Job drawing, mm, ordinate dimensions from the low corner. One solid piece. Give positions to 0.01 mm unless a question says otherwise; leave off trailing zeros. Write each loop counter-clockwise with the first axis right and the second up, starting at its lowest first coordinate (ties: lowest second). Pieces come first, ordered by that corner, then holes. Notation, with made-up numbers: M 49.5,-39 L 92.5,-39 A20 cw 92.5,-21 Z; hole C 58.5,86.25 d3. An arc over 180 degrees is marked long. Answer as CSV lines item,"result". Start each with the question number.
Item 1: Band-saw the part on B-B, the plane x = 21.5. List the corners of the cut face in (y, z).
Item 2: Band-saw the part on A-A, the plane z = 10.5. List the corners of the cut face in (x, y), then the cut area to 3 significant figures.
Item 3: Wall check: L1, parallel to Y at x = 44.5, z = 16.5; L2, parallel to Y at x = 37.5, z = 32; L3, parallel to Z at x = 46, y = 27. Give the ranges that are in metal, low to high. Write a range as from..to.
Item 4: Band-saw the part on C-C, the plane y = 10.5. List the corners of the cut face in (x, z) (3 decimals), then the cut area to 3 significant figures.
Item 5: Pin check, flat tips, straight feed: pin 1 (6 mm diameter, centred on x = 41, z = 9, fed in from -Y); pin 2 (3 mm diameter, centred on y = 10.5, z = 7.5, fed in from -X) (3 decimals). Stop position of each tip, or through.
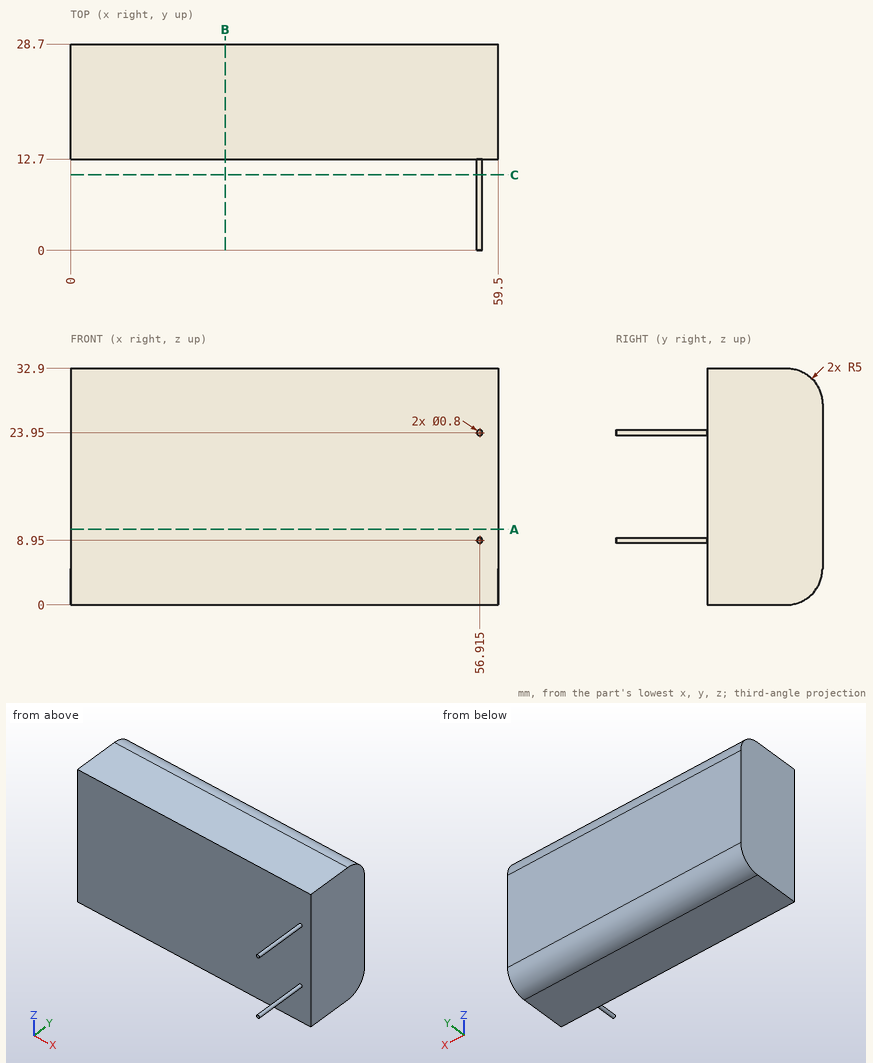
Output:
1,outline,"M 12.7,0 L 23.7,0 A5 ccw 28.7,5 L 28.7,27.9 A5 ccw 23.7,32.9 L 12.7,32.9 Z"
2,outline,"M 0,12.7 L 59.5,12.7 L 59.5,28.7 L 0,28.7 Z"
2,area,"952 mm²"
3,L1,"12.7..28.7"
3,L2,"12.7..26.56"
3,L3,"1.24..31.66"
4,outline,"C 56.915,8.95 d0.8; C 56.915,23.95 d0.8"
4,area,"1.01 mm²"
5,pin 1,"y = 12.7"
5,pin 2,"x = 56.515"
